Verification items for the finished model (mm, model axes). A direction names the side the tool comes from. Give positions to 0.01 mm unless a question says otherwise; leave off trailing zeros. Loops run counter-clockwise (first coordinate to the right, second up) from the corner with the lowest first, then second, coordinate; pieces in that order, holes last. Notation, with made-up numbers: (-37, -0.5) - (-26, -0.5) arc R21 cw to (-26, 20.5) - close; hole circle Ø1 at (-31.75, 81.5). An arc over 180 degrees is marked (long way). Use one line per item in the form item = value.
```python
from build123d import *

# Parameters (mm, degrees)
ESQUISSE1_R                  = 10
BOSS_EXTRU_1_DEPTH           = 12
ESQUISSE2_R                  = 10
BOSS_EXTRU_2_DEPTH           = 2
ESQUISSE3_R                  = 1
ENL_V_MAT_EXTRU_1_DEPTH      = 15
R_P_TITION_CIRCULAIRE1_COUNT = 25


with BuildPart() as part:
    # Esquisse1 → Boss.-Extru.1 (new body)
    with BuildSketch(Plane(origin=(0, 0, 0), x_dir=(1, 0, 0), z_dir=(0, 1, 0))):
        Circle(ESQUISSE1_R)
        with BuildLine():
            Line((2.641022529, -1.475), (-2.641022529, -1.475))
            ThreePointArc((-2.641022529, -1.475), (0, 3.025), (2.641022529, -1.475))
        make_face(mode=Mode.SUBTRACT)
    extrude(amount=BOSS_EXTRU_1_DEPTH)

    # Esquisse2 → Boss.-Extru.2 (add)
    with BuildSketch(Plane(origin=(0, 12, 0), x_dir=(1, 0, 0), z_dir=(0, 1, 0))):
        Circle(ESQUISSE2_R)
    extrude(amount=BOSS_EXTRU_2_DEPTH)

    # Esquisse3 → Enlèv. mat.-Extru.1 (cut, through all)
    with BuildSketch(Plane(origin=(0, 14, 0), x_dir=(1, 0, 0), z_dir=(0, 1, 0))):
        with Locations((0, 10.5)):
            Circle(ESQUISSE3_R)
    enl_v_mat_extru_1 = extrude(amount=-ENL_V_MAT_EXTRU_1_DEPTH, mode=Mode.SUBTRACT)

    # Répétition circulaire1: Enlèv. mat.-Extru.1 ×25 about axis
    r_p_tition_circulaire1_axis = Axis((0, 0, 0), (0, 1, 0))
    for i in range(1, R_P_TITION_CIRCULAIRE1_COUNT):
        add(enl_v_mat_extru_1.rotate(r_p_tition_circulaire1_axis, i * 360 / R_P_TITION_CIRCULAIRE1_COUNT), mode=Mode.SUBTRACT)


solid = part.part
```
1. Section check A-A, the plane x = 0. Record the cut outline in (y, z) (3 decimals), then the cut area to 3 significant figures.
Result set:
outline = (0, -9.5) - (14, -9.5) - (14, 10) - (0, 10) - (0, 1.475) - (12, 1.475) - (12, -3.025) - (0, -3.025) - close
area = 219 mm²
2. Scan lines: probe 1 along Z at (x, y) = (0, 3) (3 decimals); probe 2 along X at (y, z) = (5.5, 0) (3 decimals); probe 3 along Z at (x, y) = (0.5, 6.5) (3 decimals). Record each from-to range of solid material in increasing order.
Result set:
probe_1 = -9.5 to -3.025, 1.475 to 10
probe_2 = -9.727 to -3.025, 3.025 to 9.727
probe_3 = -9.634 to -2.983, 1.475 to 9.839
3. Draft check along Z on faces 3 (the cylindrical face through (9.824, 6.902, -1.868)), 4 (the cylindrical face through (-7.31, 7.1, 6.07)), 5 (the cylindrical face through (9.98, 6.9, 0.63)). Enter one of: released by +Z, released by -Z, zero draft, split by the parting line, or undercut.
Result set:
face_3 = released by -Z
face_4 = undercut
face_5 = released by +Z
4. Section check D-D, the plane z = -3.5. Record the cut outline in (x, y), then the cut area to 3 significant figures.
Result set:
outline = (-9.02, 0) - (9.02, 0) - (9.02, 14) - (-9.02, 14) - close
area = 253 mm²
5. Depth check by flat-ended pin: pin 1 Ø2 at (x, y) = (-3.5, 10) entering from -Z; pin 2 Ø6 at (y, z) = (1.5, -4.5) entering from -X; pin 3 Ø8 at (y, z) = (8, -6.5) entering from +X. Enter the tip coordinate at first touch or a pass-through.
Result set:
pin_1 = -9.44
pin_2 = -9.89
pin_3 = 9.32
6. Section check B-B, the plane z = -1. Record the cut outline in (x, y).
Result set:
outline = (-9.54, 0) - (-2.85, 0) - (-2.85, 12) - (2.85, 12) - (2.85, 0) - (9.54, 0) - (9.54, 14) - (-9.54, 14) - close
7. Section check C-C, the plane x = 3.75. Record the cut outline in (y, z).
Result set:
outline = (0, -9.27) - (14, -9.27) - (14, 8.77) - (0, 8.77) - close
8. Tool access check on faces 1 (the flat face through (0, 12, 0)), 2 (the cylindrical face through (-3.48, 7.1, 8.84)). Record the directions out of +Z, -Z, +X, -X, +Y, -Y that give a thin tool (end or side, any length) a straight path to the whole face; none if there is none.
Result set:
face_1 = -Y
face_2 = +Z, +Y, -Y
